```python
from build123d import *

# Parameters (mm, degrees)
BOSS_EXTRUDE2_DEPTH     = 20
CUT_EXTRUDE1_DEPTH      = 20
SKETCH7_W               = 242.556539121
SKETCH7_H               = 25
BOSS_EXTRUDE3_DEPTH     = 5
SKETCH8_W               = 242.556539121
SKETCH8_H               = 25
BOSS_EXTRUDE4_DEPTH     = 5
CUT_EXTRUDE2_DEPTH      = 473.361090692
CUT_EXTRUDE2_DEPTH_BACK = 473.361090692
SKETCH11_W              = 30
SKETCH11_H              = 25
BOSS_EXTRUDE5_DEPTH     = 5
SKETCH13_W              = 30
SKETCH13_H              = 25
BOSS_EXTRUDE6_DEPTH     = 5
SKETCH14_R              = 5
CUT_EXTRUDE3_DEPTH      = 473.361090692
BOSS_EXTRUDE7_DEPTH     = 5
BOSS_EXTRUDE8_START     = -5
BOSS_EXTRUDE8_DEPTH     = 5
SKETCH19_R              = 5
CUT_EXTRUDE4_DEPTH      = 473.361090692


with BuildPart() as part:
    # Sketch5 → Boss-Extrude2 (new body)
    with BuildSketch(Plane(origin=(0, 0, 0), x_dir=(1, 0, 0), z_dir=(0, 1, 0))):
        with BuildLine():
            Line((-180, 250), (180, 250))
            ThreePointArc((180, 250), (194.142135624, 244.142135624), (200, 230))
            Line((200, 230), (200, -230))
            ThreePointArc((200, -230), (194.142135624, -244.142135624), (180, -250))
            Line((180, -250), (-180, -250))
            ThreePointArc((-180, -250), (-194.142135624, -244.142135624), (-200, -230))
            Line((-200, -230), (-200, 230))
            ThreePointArc((-200, 230), (-194.142135624, 244.142135624), (-180, 250))
        make_face()
    extrude(amount=BOSS_EXTRUDE2_DEPTH)

    # Sketch6 → Cut-Extrude1 (cut)
    with BuildSketch(Plane(origin=(0, 20, 0), x_dir=(1, 0, 0), z_dir=(0, 1, 0))):
        with BuildLine():
            Line((-175, -245), (175, -245))
            ThreePointArc((175, -245), (189.142135624, -239.142135624), (195, -225))
            Line((195, -225), (195, 225))
            ThreePointArc((195, 225), (189.142135624, 239.142135624), (175, 245))
            Line((175, 245), (-175, 245))
            ThreePointArc((-175, 245), (-189.142135624, 239.142135624), (-195, 225))
            Line((-195, 225), (-195, -225))
            ThreePointArc((-195, -225), (-189.142135624, -239.142135624), (-175, -245))
        make_face()
    extrude(amount=-CUT_EXTRUDE1_DEPTH, mode=Mode.SUBTRACT)

    # Sketch7 → Boss-Extrude3 (add)
    with BuildSketch(Plane(origin=(200, 0, 0), x_dir=(0, 0, -1), z_dir=(1, 0, 0))):
        with Locations((108.72173044, -12.5)):
            Rectangle(SKETCH7_W, SKETCH7_H)
    extrude(amount=-BOSS_EXTRUDE3_DEPTH)

    # Sketch8 → Boss-Extrude4 (add)
    with BuildSketch(Plane.ZY.offset(200)):
        with Locations((-108.72173044, -12.5)):
            Rectangle(SKETCH8_W, SKETCH8_H)
    extrude(amount=-BOSS_EXTRUDE4_DEPTH)

    # Sketch10 → Cut-Extrude2 (cut, two sides: drawn at the far end of the back side and taken through both)
    with BuildSketch(Plane(origin=(200, 0, 0), x_dir=(0, 0, -1), z_dir=(1, 0, 0)).offset(-CUT_EXTRUDE2_DEPTH_BACK)):
        with BuildLine():
            Line((214.975112076, -7.5), (2.443460879, -7.5))
            ThreePointArc((2.443460879, -7.5), (-2.556539121, -12.5), (2.443460879, -17.5))
            Line((2.443460879, -17.5), (214.975112076, -17.5))
            ThreePointArc((214.975112076, -17.5), (219.975112076, -12.5), (214.975112076, -7.5))
        make_face()
    extrude(amount=CUT_EXTRUDE2_DEPTH + CUT_EXTRUDE2_DEPTH_BACK, mode=Mode.SUBTRACT)

    # Sketch11 → Boss-Extrude5 (add)
    with BuildSketch(Plane(origin=(200, 0, 0), x_dir=(0, 0, -1), z_dir=(1, 0, 0))):
        with Locations((-215, -12.5)):
            Rectangle(SKETCH11_W, SKETCH11_H)
    extrude(amount=-BOSS_EXTRUDE5_DEPTH)

    # Sketch13 → Boss-Extrude6 (add)
    with BuildSketch(Plane.ZY.offset(200)):
        with Locations((215, -12.5)):
            Rectangle(SKETCH13_W, SKETCH13_H)
    extrude(amount=-BOSS_EXTRUDE6_DEPTH)

    # Sketch14 → Cut-Extrude3 (cut, through all)
    with BuildSketch(Plane.ZY.offset(200)):
        with Locations((215, -12.5)):
            Circle(SKETCH14_R)
    extrude(amount=-CUT_EXTRUDE3_DEPTH, mode=Mode.SUBTRACT)

    # Sketch16 → Boss-Extrude7 (add)
    with BuildSketch(Plane.ZY.offset(200)):
        with BuildLine():
            Line((-67.443460879, -17.5), (-2.443460879, -17.5))
            ThreePointArc((-2.443460879, -17.5), (2.556539121, -12.5), (-2.443460879, -7.5))
            Line((-2.443460879, -7.5), (-67.443460879, -7.5))
            Line((-67.443460879, -7.5), (-67.443460879, -17.5))
        make_face()
    extrude(amount=-BOSS_EXTRUDE7_DEPTH)

    # Sketch17 → Boss-Extrude8 (add)
    with BuildSketch(Plane(origin=(200, 0, 0), x_dir=(0, 0, -1), z_dir=(1, 0, 0)).offset(BOSS_EXTRUDE8_START)):
        with BuildLine():
            Line((67.443460879, -17.5), (67.443460879, -7.5))
            Line((67.443460879, -7.5), (2.443460879, -7.5))
            ThreePointArc((2.443460879, -7.5), (-2.556539121, -12.5), (2.443460879, -17.5))
            Line((2.443460879, -17.5), (67.443460879, -17.5))
        make_face()
    extrude(amount=BOSS_EXTRUDE8_DEPTH)

    # Sketch19 → Cut-Extrude4 (cut, through all)
    with BuildSketch(Plane(origin=(200, 0, 0), x_dir=(0, 0, -1), z_dir=(1, 0, 0))):
        with Locations((221.779838072, 10)):
            Circle(SKETCH19_R)
    extrude(amount=-CUT_EXTRUDE4_DEPTH, mode=Mode.SUBTRACT)


solid = part.part
```
Input: part model. Units: mm. Frame: model coordinates. A direction names the side the tool comes from. Give positions to 0.01 mm unless a question says otherwise; leave off trailing zeros. Order: outer loops, then holes, each group sorted by start corner. A loop starts at its lowest first (then second) coordinate and runs counter-clockwise, first axis right, second up. Notation, with made-up numbers: (46.5, 50.25) - (71.5, 50.25) arc R26 cw to (71.5, 86.25) - close; hole circle Ø2 at (38, 82). An arc over 180 degrees is marked (long way). Use a Markdown table: item, result.
(1) Draft query along Y for faces 3 (the cylindrical face through (-197.42, 11.5, -226.55)), 4 (the cylindrical face through (-194.297, 9.86, -243.986)). Return one class per face: released by +Y, released by -Y, zero draft, split by the parting line, or undercut.
Computed values:
| item | result |
|---|---|
| face 3 | undercut |
| face 4 | zero draft |
(2) Line query: line 1 (X direction, y = -6.5, z = -122); line 2 (Z direction, x = 60, y = 16.5); line 3 (Y direction, x = -197, z = 215). Output: solid intervals per line, ascending. Write a range as from..to.
Computed values:
| item | result |
|---|---|
| line 1 | x = -200..-195, 195..200 |
| line 2 | z = -250..-245, 245..250 |
| line 3 | y = -25..-17.5, -7.5..20 |
(3) Section query B-B (x = -108.5). Output: boundary loops of the cut face in (y, z).
Computed values:
| item | result |
|---|---|
| outline | (0, -250) - (20, -250) - (20, -245) - (0, -245) - close; (0, 245) - (20, 245) - (20, 250) - (0, 250) - close |
(4) Section query A-A (z = -125). Output: boundary loops of the cut face in (x, y), then the cut area to 3 significant figures.
Computed values:
| item | result |
|---|---|
| outline | (-200, -25) - (-195, -25) - (-195, -17.5) - (-200, -17.5) - close; (-200, -7.5) - (-195, -7.5) - (-195, 20) - (-200, 20) - close; (195, -25) - (200, -25) - (200, -17.5) - (195, -17.5) - close; (195, -7.5) - (200, -7.5) - (200, 20) - (195, 20) - close |
| area | 350 mm2 |
(5) Section query C-C (z = 70.5). Output: boundary loops of the cut face in (x, y), then the cut area to 3 significant figures.
Computed values:
| item | result |
|---|---|
| outline | (-200, 0) - (-195, 0) - (-195, 20) - (-200, 20) - close; (195, 0) - (200, 0) - (200, 20) - (195, 20) - close |
| area | 200 mm2 |
(6) Access query for faces 1 (the cylindrical face through (-188.986, 10.14, -239.297)), 2 (the flat face through (3, 10, 250)). Directions: +Z, -Z, +X, -X, +Y, -Y. A direction counts if a zero-diameter tool reaches every point of the face in a straight line with its end or side. Return the directions, or none.
Computed values:
| item | result |
|---|---|
| face 1 | +Y, -Y |
| face 2 | +Z, +X, -X, +Y, -Y |
(7) Pin query (flat end, axial travel): pin 1 (2.5 mm diameter, centred on x = 197.5, y = -11, fed in from +Z); pin 2 (10 mm diameter, centred on y = -13.5, z = -131.5, fed in from +X); pin 3 (4 mm diameter, centred on x = -197.5, z = 93, fed in from -Y); pin 4 (2.5 mm diameter, centred on x = -197, y = -12.5, fed in from -Z). Return the tip coordinate at first contact, or that it passes through.
Computed values:
| item | result |
|---|---|
| pin 1 | stops at z = 230 |
| pin 2 | stops at x = 200 |
| pin 3 | stops at y = 0 |
| pin 4 | stops at z = -230 |
